The model under review builds one solid part; all positions refer to its coordinate system, in mm. A direction names the side the tool comes from. Round coordinates to 2 decimals unless told otherwise and drop trailing zeros. Loops run counter-clockwise (first coordinate to the right, second up) from the corner with the lowest first, then second, coordinate; pieces in that order, holes last. Notation, with made-up numbers: (45.25, -25) -> (57.25, -25) arc R29 cw to (57.25, -2) -> close; hole circle Ø8 at (-19, 16.25). An arc over 180 degrees is marked (long way). Return JSON: item names as keys, results as strings. Group by question number.
```python
from build123d import *

# Parameters (mm, degrees)
F0_R     = 13
F1_DEPTH = 3
F0_R_2   = 16
F2_DEPTH = 8
F3_R     = 3


with BuildPart() as f1:
    # F0 (on Top) → F1 (new body)
    with BuildSketch(Plane.XY):
        Circle(F0_R)
    extrude(amount=F1_DEPTH)

    # F0 (on Top) → F2 (join)
    with BuildSketch(Plane.XY):
        Circle(F0_R_2)
        Circle(F0_R, mode=Mode.SUBTRACT)
    extrude(amount=F2_DEPTH)

    # F3
    f3_edges = [f1.edges().sort_by_distance(p)[0] for p in [
        (-16, 0, 0),
    ]]
    fillet(f3_edges, radius=F3_R)


solid = f1.part
```
1. Wall thickness on line 1 (Y direction, x = 0, z = 4.65); line 2 (X direction, y = 11, z = 3.5); line 3 (Y direction, x = -5, z = 4.25): over which ranges is each line inside the solid? List them lowest first.
2. Tool access review of faces 4 (the face through (0, 0, 0)), 5 (the face through (0, 0, 3)): name each direction out of +Z, -Z, +X, -X, +Y, -Y from which nothing blocks a thin tool from reaching the whole face with its end or side.
3. For P1, Ø1, axis at x = 10, z = 1.5, coming from the +Y side; P2, Ø8, axis at x = 1.5, y = -6, coming from the +Z side; P3, Ø2, axis at x = 12, z = 2.5, coming from the -Y side, all flat-tipped, find the tip position at first contact; note any pin that passes through.
4. Draft analysis for pull direction Y (two halves, no side actions). For faces 1 (the face through (-10.316, -7.91, 5.465)), 2 (the face through (-3.47, -15.62, 5.46)), 3 (the face through (-1.3, 13.1, 8)), state which applies: pulls with the +Y half, pulls with the -Y half, needs draft (parallel to the pull), parting line crosses it, or undercut.
5. We need section D-D, the plane z = 1.75. Write out the cut boundary in (x, y), then the cut area to 3 significant figures.
6. We need section C-C, the plane z = 5.25. Write out the cut boundary in (x, y).
7. We need section A-A, the plane y = 0. Write out the cut boundary in (x, z).
Check sheet entries:
{
 "1": {"line 1": "y = -16 to -13, 13 to 16", "line 2": "x = -11.62 to -6.93, 6.93 to 11.62", "line 3": "y = -15.2 to -12, 12 to 15.2"},
 "2": {"face 4": "-Z, +X, -X, +Y, -Y", "face 5": "+Z"},
 "3": {"P1": "stops at y = 12.49", "P2": "stops at z = 3", "P3": "stops at y = -11.58"},
 "4": {"face 1": "undercut", "face 2": "parting line crosses it", "face 3": "needs draft"},
 "5": {"outline": "circle Ø31.45 at (0, 0)", "area": "777 mm²"},
 "6": {"outline": "circle Ø32 at (0, 0); hole circle Ø26 at (0, 0)"},
 "7": {"outline": "(-16, 3) arc R3 ccw to (-13, 0) -> (13, 0) arc R3 ccw to (16, 3) -> (16, 8) -> (13, 8) -> (13, 3) -> (-13, 3) -> (-13, 8) -> (-16, 8) -> close"}
}
